The listing builds one solid part. Answer for the finished solid, in the listing's coordinates (mm). Face numbers are marked on the shaded views. Coordinates: 2 decimals unless noted, no trailing zeros. Write each loop counter-clockwise with the first axis right and the second up, starting at its lowest first coordinate (ties: lowest second). Pieces come first, ordered by that corner, then holes.
```python
from build123d import *

# Parameters (mm, degrees)
SKETCH1_W            = 43
SKETCH1_H            = 20
BOSS_EXTRUDE1_DEPTH  = 1.6
SKETCH2_R            = 8
BOSS_EXTRUDE2_DEPTH  = 14
SKETCH3_R            = 6.893962295
CUT_EXTRUDE1_DEPTH   = 2
FILLET1_R            = 1
FILLET2_R            = 1
FILLET1_OF_MIRROR1_R = 1
FILLET2_OF_MIRROR1_R = 1
BOSS_EXTRUDE3_DEPTH  = 2
SKETCH5_W            = 0.6
SKETCH5_H            = 0.6
BOSS_EXTRUDE4_DEPTH  = 6
CHAMFER1_SIZE        = 0.1
CHAMFER2_SIZE        = 0.1
CUT_EXTRUDE2_REACH   = 3.6
SKETCH6_R            = 1.05


with BuildPart() as part:
    # Sketch1 → Boss-Extrude1 (new body)
    with BuildSketch(Plane(origin=(0, 0, 0), x_dir=(1, 0, 0), z_dir=(0, 1, 0))):
        with Locations((21.5, 10)):
            Rectangle(SKETCH1_W, SKETCH1_H)
    extrude(amount=BOSS_EXTRUDE1_DEPTH)

    # Sketch2 → Boss-Extrude2 (add)
    with BuildSketch(Plane(origin=(0, 1.6, 0), x_dir=(1, 0, 0), z_dir=(0, 1, 0))):
        with Locations((10, 10)):
            Circle(SKETCH2_R)
    boss_extrude2 = extrude(amount=BOSS_EXTRUDE2_DEPTH)

    # Sketch3 → Cut-Extrude1 (cut)
    with BuildSketch(Plane(origin=(0, 15.6, 0), x_dir=(1, 0, 0), z_dir=(0, 1, 0))):
        with Locations((10, 10)):
            Circle(SKETCH3_R)
    cut_extrude1 = extrude(amount=-CUT_EXTRUDE1_DEPTH, mode=Mode.SUBTRACT)

    # Fillet1
    fillet1_edges = [part.edges().sort_by_distance(p)[0] for p in [
        (2, 15.6, -10),
    ]]
    fillet(fillet1_edges, radius=FILLET1_R)

    # Fillet2
    fillet2_edges = [part.edges().sort_by_distance(p)[0] for p in [
        (3.106037705, 13.6, -10),
    ]]
    fillet(fillet2_edges, radius=FILLET2_R)

    # Mirror1: Boss-Extrude2, Cut-Extrude1 across plane
    add(boss_extrude2.mirror(Plane(origin=(21.5, 0, 0), x_dir=(0, 0, 1), z_dir=(1, 0, 0))))
    add(cut_extrude1.mirror(Plane(origin=(21.5, 0, 0), x_dir=(0, 0, 1), z_dir=(1, 0, 0))), mode=Mode.SUBTRACT)

    # Fillet1 of Mirror1
    fillet1_of_mirror1_edges = [part.edges().sort_by_distance(p)[0] for p in [
        (41, 15.6, -10),
    ]]
    fillet(fillet1_of_mirror1_edges, radius=FILLET1_OF_MIRROR1_R)

    # Fillet2 of Mirror1
    fillet2_of_mirror1_edges = [part.edges().sort_by_distance(p)[0] for p in [
        (39.893962295, 13.6, -10),
    ]]
    fillet(fillet2_of_mirror1_edges, radius=FILLET2_OF_MIRROR1_R)

    # Sketch4 → Boss-Extrude3 (add)
    with BuildSketch(Plane(origin=(0, 1.6, 0), x_dir=(1, 0, 0), z_dir=(0, 1, 0))):
        Polygon((21.5, 0), (18.65, 0), (18.65, 2.7), (24.35, 2.7), (24.35, 0), align=None)
    extrude(amount=BOSS_EXTRUDE3_DEPTH)

    # Sketch5 → Boss-Extrude4 (add)
    with BuildSketch(Plane.XY):
        with Locations((19.322458837, 2.6)):
            Rectangle(SKETCH5_W, SKETCH5_H)
        with Locations((20.752458837, 2.6)):
            Rectangle(SKETCH5_W, SKETCH5_H)
        with Locations((22.182458837, 2.6)):
            Rectangle(SKETCH5_W, SKETCH5_H)
        with Locations((23.612458837, 2.6)):
            Rectangle(SKETCH5_W, SKETCH5_H)
    extrude(amount=BOSS_EXTRUDE4_DEPTH)

    # Chamfer1
    chamfer1_edges = [part.edges().sort_by_distance(p)[0] for p in [
        (19.622458837, 2.3, 3),
        (19.622458837, 2.9, 3),
        (19.022458837, 2.9, 3),
        (19.022458837, 2.3, 3),
        (19.622458837, 2.6, 6),
        (19.322458837, 2.9, 6),
        (19.022458837, 2.6, 6),
        (19.322458837, 2.3, 6),
        (21.052458837, 2.9, 3),
        (20.452458837, 2.9, 3),
        (20.452458837, 2.3, 3),
        (21.052458837, 2.3, 3),
        (20.752458837, 2.9, 6),
        (20.452458837, 2.6, 6),
        (20.752458837, 2.3, 6),
        (21.052458837, 2.6, 6),
        (22.482458837, 2.9, 3),
        (21.882458837, 2.9, 3),
        (21.882458837, 2.3, 3),
        (22.482458837, 2.3, 3),
        (22.182458837, 2.9, 6),
        (21.882458837, 2.6, 6),
        (22.182458837, 2.3, 6),
        (22.482458837, 2.6, 6),
        (23.912458837, 2.9, 3),
        (23.312458837, 2.9, 3),
        (23.312458837, 2.3, 3),
        (23.912458837, 2.3, 3),
        (23.612458837, 2.9, 6),
        (23.312458837, 2.6, 6),
        (23.612458837, 2.3, 6),
        (23.912458837, 2.6, 6),
    ]]
    chamfer(chamfer1_edges, length=CHAMFER1_SIZE)

    # Chamfer2
    chamfer2_edges = [part.edges().sort_by_distance(p)[0] for p in [
        (21.5, 3.6, 0),
        (24.35, 3.6, -1.35),
        (21.5, 3.6, -2.7),
        (18.65, 3.6, -1.35),
    ]]
    chamfer(chamfer2_edges, length=CHAMFER2_SIZE)

    # Sketch6 → Cut-Extrude2 (cut, up to next)
    with BuildSketch(Plane(origin=(0, 1.6, 0), x_dir=(1, 0, 0), z_dir=(0, 1, 0)), mode=Mode.PRIVATE) as cut_extrude2_sk1:
        with Locations((1.5, 18.5)):
            Circle(SKETCH6_R)
    cut_extrude2_tool1 = extrude(cut_extrude2_sk1.sketch, amount=-CUT_EXTRUDE2_REACH, mode=Mode.PRIVATE) & part.part
    add(cut_extrude2_tool1.solids().sort_by_distance((1.5, 1.6, -18.5))[0], mode=Mode.SUBTRACT)
    # Sketch6 → Cut-Extrude2 (cut, up to next)
    with BuildSketch(Plane(origin=(0, 1.6, 0), x_dir=(1, 0, 0), z_dir=(0, 1, 0)), mode=Mode.PRIVATE) as cut_extrude2_sk2:
        with Locations((1.5, 1.5)):
            Circle(SKETCH6_R)
    cut_extrude2_tool2 = extrude(cut_extrude2_sk2.sketch, amount=-CUT_EXTRUDE2_REACH, mode=Mode.PRIVATE) & part.part
    add(cut_extrude2_tool2.solids().sort_by_distance((1.5, 1.6, -1.5))[0], mode=Mode.SUBTRACT)
    # Sketch6 → Cut-Extrude2 (cut, up to next)
    with BuildSketch(Plane(origin=(0, 1.6, 0), x_dir=(1, 0, 0), z_dir=(0, 1, 0)), mode=Mode.PRIVATE) as cut_extrude2_sk3:
        with Locations((41.5, 1.5)):
            Circle(SKETCH6_R)
    cut_extrude2_tool3 = extrude(cut_extrude2_sk3.sketch, amount=-CUT_EXTRUDE2_REACH, mode=Mode.PRIVATE) & part.part
    add(cut_extrude2_tool3.solids().sort_by_distance((41.5, 1.6, -1.5))[0], mode=Mode.SUBTRACT)
    # Sketch6 → Cut-Extrude2 (cut, up to next)
    with BuildSketch(Plane(origin=(0, 1.6, 0), x_dir=(1, 0, 0), z_dir=(0, 1, 0)), mode=Mode.PRIVATE) as cut_extrude2_sk4:
        with Locations((41.5, 18.5)):
            Circle(SKETCH6_R)
    cut_extrude2_tool4 = extrude(cut_extrude2_sk4.sketch, amount=-CUT_EXTRUDE2_REACH, mode=Mode.PRIVATE) & part.part
    add(cut_extrude2_tool4.solids().sort_by_distance((41.5, 1.6, -18.5))[0], mode=Mode.SUBTRACT)


solid = part.part
```
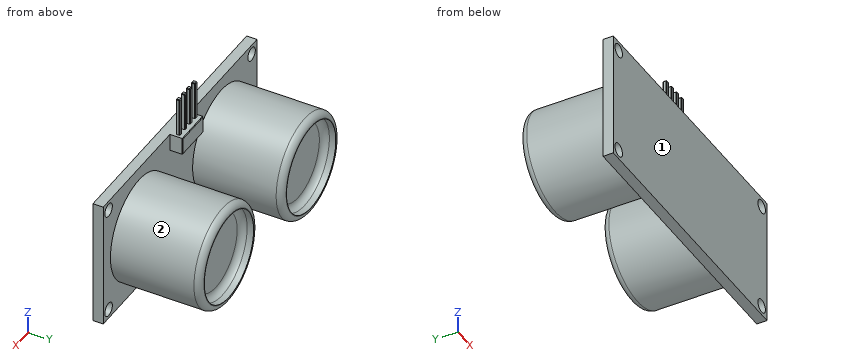
(1) For a pull along X with two mould halves and no side action, classify the marked faces 1 and 2 as pulls with the +X half, pulls with the -X half, needs draft (parallel to the pull), parting line crosses it, or undercut.
(2) Find the intervals of material crossed by probe 1 along X at (y, z) = (0.55, -1.5); probe 2 along Z at (x, y) = (41.5, 0.65); probe 3 along X at (y, z) = (2.5, 4.5), in increasing order.
(3) Section B-B, the plane x = 1.5 is taken. Write down the section's boundary in (y, z), plus the area to 3 significant figures.
(4) Section A-A, the plane z = -1.5 is taken. Write down the section's boundary in (x, y), plus the area to 3 significant figures.
(5) Each of these flat-tipped pins is pushed along its axis until it touches: pin 1 (2.5 mm diameter, centred on x = 1.5, z = -18.5, fed in from +Y); pin 2 (1.7 mm diameter, centred on x = 1.5, z = -1.5, fed in from +Y); pin 3 (5 mm diameter, centred on x = 11, y = 10.5, fed in from -Z); pin 4 (1 mm diameter, centred on y = 5, z = -4.5, fed in from +X) (3 decimals). Where does it stop, or does it pass through?
(6) Section D-D, the plane y = 6.25 is taken. Write down the section's boundary in (x, z), plus the area to 3 significant figures.
(7) Section C-C, the plane z = 3 is taken. State how many separate pieces and enclosed holes the cut face has, plus the area to 3 significant figures.
Solution:
1. face 1: needs draft
1. face 2: undercut
2. probe 1: x = 0 to 0.45, 2.55 to 40.45, 42.55 to 43
2. probe 2: z = -20 to -19.55, -17.45 to -2.55, -0.45 to 0
2. probe 3: x = 19.02 to 19.62, 20.45 to 21.05, 21.88 to 22.48, 23.31 to 23.91
3. outline: (0, -20) - (1.6, -20) - (1.6, -19.55) - (0, -19.55) - close; (0, -17.45) - (1.6, -17.45) - (1.6, -2.55) - (0, -2.55) - close; (0, -0.45) - (1.6, -0.45) - (1.6, 0) - (0, 0) - close
3. area: 25.3 mm2
4. outline: (0, 0) - (0.45, 0) - (0.45, 1.6) - (0, 1.6) - close; (2.55, 0) - (40.45, 0) - (40.45, 1.6) - (24.35, 1.6) - (24.35, 3.5) - (24.25, 3.6) - (18.75, 3.6) - (18.65, 3.5) - (18.65, 1.6) - (2.55, 1.6) - close; (42.55, 0) - (43, 0) - (43, 1.6) - (42.55, 1.6) - close
4. area: 73.5 mm2
5. pin 1: stops at y = 1.6
5. pin 2: passes through
5. pin 3: stops at z = -18
5. pin 4: stops at x = 39.245
6. outline: circle Ø16 at (10, -10); circle Ø16 at (33, -10)
6. area: 402 mm2
7. separate pieces: 4
7. enclosed holes: 0
7. area: 1.36 mm2
